Build history of the part. All positions in model axes, mm. Face numbers are marked on the shaded views. Round coordinates to 2 decimals unless told otherwise and drop trailing zeros. Order: outer loops, then holes, each group sorted by start corner. A loop starts at its lowest first (then second) coordinate and runs counter-clockwise, first axis right, second up. Notation, with made-up numbers: M 20,34.25 L 61,34.25 A10 ccw 61,38.25 Z; hole C 83.5,8.5 d7. An arc over 180 degrees is marked long. One line per item, written item: value. Start each with the question number.
Item 1: Band-saw the part on B-B, the plane x = -10. Write the cut outline in (y, z), then the cut area to 3 significant figures.
Item 2: Probe L1, parallel to Y at x = -26, z = 0.7; L2, parallel to Y at x = 0.5, z = 2; L3, parallel to X at y = -2.75, z = 1.75. List the from-to ranges inside material, lowest first.
Item 3: Band-saw the part on C-C, the plane z = 1.1. Write the cut outline in (x, y), then the cut area to 3 significant figures.
Item 4: Band-saw the part on A-A, the plane y = 0. Give the number of separate pieces and of enclosed holes in the cut face, then the cut area to 3 significant figures.
Item 5: Band-saw the part on D-D, the plane y = -2.5. Write the cut outline in (x, z).
Item 6: Two-plate mould, pull along Y, no slides. Class the marked faces 1, 2 and 3: +Y half, -Y half, draft (parallel to the pull), parting line (faces both ways), or undercut.
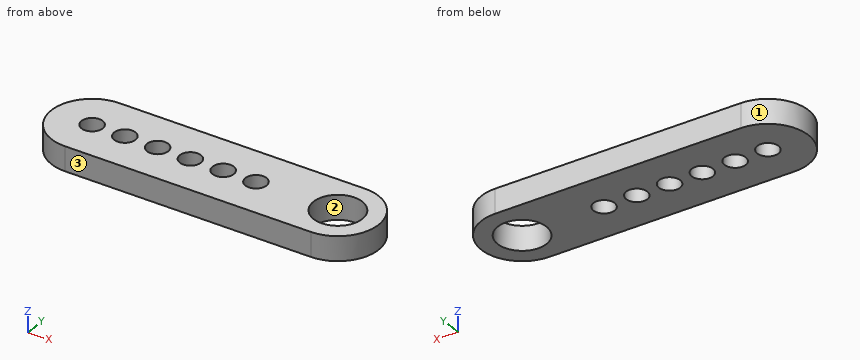
```python
from build123d import *

# Parameters (mm, degrees)
ESQUISSE1_R        = 1.305103473
ESQUISSE1_R_2      = 3
BOSS_EXTRU_1_DEPTH = 3


with BuildPart() as part:
    # Esquisse1 → Boss.-Extru.1 (new body)
    with BuildSketch(Plane.XY):
        with BuildLine():
            Line((-30, -5), (0, -5))
            ThreePointArc((0, -5), (5, 0), (0, 5))
            Line((0, 5), (-30, 5))
            ThreePointArc((-30, 5), (-35, 0), (-30, -5))
        make_face()
        with Locations((-30, 0)):
            Circle(ESQUISSE1_R, mode=Mode.SUBTRACT)
        with Locations((-26, 0)):
            Circle(ESQUISSE1_R, mode=Mode.SUBTRACT)
        with Locations((-22, 0)):
            Circle(ESQUISSE1_R, mode=Mode.SUBTRACT)
        with Locations((-18, 0)):
            Circle(ESQUISSE1_R, mode=Mode.SUBTRACT)
        with Locations((-14, 0)):
            Circle(ESQUISSE1_R, mode=Mode.SUBTRACT)
        with Locations((-10, 0)):
            Circle(ESQUISSE1_R, mode=Mode.SUBTRACT)
        Circle(ESQUISSE1_R_2, mode=Mode.SUBTRACT)
    extrude(amount=BOSS_EXTRU_1_DEPTH)


solid = part.part
```
Output:
1. outline: M -5,0 L -1.31,0 L -1.31,3 L -5,3 Z; M 1.31,0 L 5,0 L 5,3 L 1.31,3 Z
1. area: 22.2 mm²
2. L1: y = -5 to -1.31, 1.31 to 5
2. L2: y = -4.97 to -2.96, 2.96 to 4.97
2. L3: x = -34.18 to -1.2, 1.2 to 4.18
3. outline: M -30,-5 L 0,-5 A5 ccw 0,5 L -30,5 A5 ccw Z; hole C -30,0 d2.61; hole C -26,0 d2.61; hole C -22,0 d2.61; hole C -18,0 d2.61; hole C -14,0 d2.61; hole C -10,0 d2.61; hole C 0,0 d6
3. area: 318 mm²
4. separate pieces: 8
4. enclosed holes: 0
4. area: 55.0 mm²
5. outline: M -34.33,0 L -1.66,0 L -1.66,3 L -34.33,3 Z; M 1.66,0 L 4.33,0 L 4.33,3 L 1.66,3 Z
6. face 1: parting line
6. face 2: undercut
6. face 3: -Y half
